```python
from build123d import *

# Parameters (mm, degrees)
SKETCH1_W            = 1180
SKETCH1_H            = 168
BASE_FLANGE1_DEPTH   = 12
EDGE_FLANGE1_START   = -590
EDGE_FLANGE1_DEPTH   = 1180
EDGE_FLANGE1_2_DEPTH = 1180


# Read off the part's stored shape, not the designer's step: Edge-Flange1
# Sheet-metal steps are written as plain solids
with BuildPart() as part:
    # Sketch1 → Base-Flange1 (new body)
    with BuildSketch(Plane(origin=(0, 0, 0), x_dir=(1, 0, 0), z_dir=(0, 1, 0))):
        Rectangle(SKETCH1_W, SKETCH1_H)
    extrude(amount=-BASE_FLANGE1_DEPTH)

    # Edge-Flange1 outline → Edge-Flange1 (cut)
    with BuildSketch(Plane.YZ.offset(EDGE_FLANGE1_START)):
        with BuildLine():
            Line((0, -84), (-8.382685902, -69.480762114))
            ThreePointArc((-8.382685902, -69.480762114), (-11.07999731, -62.968876332), (-12, -55.980762114))
            Line((-12, -55.980762114), (-12, -84))
            Line((-12, -84), (0, -84))
        make_face()
    extrude(amount=EDGE_FLANGE1_DEPTH, mode=Mode.SUBTRACT)

    # Edge-Flange1 2 outline → Edge-Flange1 2 (add)
    with BuildSketch(Plane.YZ.offset(EDGE_FLANGE1_START)):
        with BuildLine():
            Line((0, -55.980762114), (0, -84))
            Line((0, -84), (3, -89.196152423))
            Line((3, -89.196152423), (13.392304845, -83.196152423))
            Line((13.392304845, -83.196152423), (2.009618943, -63.480762114))
            ThreePointArc((2.009618943, -63.480762114), (0.511112606, -59.86304779), (0, -55.980762114))
        make_face()
    extrude(amount=EDGE_FLANGE1_2_DEPTH)


solid = part.part
```
Geometry check sheet. Reference: the model listing, model coordinates, mm. A direction names the side the tool comes from. Give positions to 0.01 mm unless a question says otherwise; leave off trailing zeros. Write each loop counter-clockwise with the first axis right and the second up, starting at its lowest first coordinate (ties: lowest second). Pieces come first, ordered by that corner, then holes.
1) Section check C-C, the plane y = 8.75. Record the boundary of the cut face in (x, z).
2) Access from +Z, -Z, +X, -X, +Y, -Y to the whole of each face (thin tool, end or side, straight path). Record for faces 1 (the flat face through (-8, 0, 13)), 2 (the flat face through (-8, -12, 13)).
3) Gauge pin test, flat ends, axial feed: pin 1 (5 mm diameter, centred on x = -184.5, y = 0.5, fed in from +Z); pin 2 (2 mm diameter, centred on x = -399, z = -34.5, fed in from +Y); pin 3 (3 mm diameter, centred on x = -280.5, y = 7.5, fed in from -Z). Record the tip position at first contact, or that the pin passes through.
4) Section check B-B, the plane z = 57. Record the boundary of the cut face in (x, y).
5) Material ranges on L1, parallel to Y at x = 530, z = 69; L2, parallel to Z at x = -482.5, y = 7; L3, parallel to Z at x = 65, y = 9.25, recorded low to high.
6) Section check A-A, the plane x = -275. Record the boundary of the cut face in (y, z), and give its area (3 significant figures).
Computed:
1. outline: (-590, -85.88) - (590, -85.88) - (590, -75.16) - (-590, -75.16) - close
2. face 1: +Z, +X, -X, +Y
2. face 2: +Z, -Z, +X, -X, -Y
3. pin 1: stops at z = 84
3. pin 2: stops at y = 0
3. pin 3: stops at z = -87.46
4. outline: (-590, -12) - (590, -12) - (590, 0) - (-590, 0) - close
5. L1: y = -12 to 0
5. L2: z = -86.89 to -72.12
5. L3: z = -85.59 to -76.02
6. outline: (-12, -55.98) arc R27 ccw to (-8.38, -69.48) - (3, -89.2) - (13.39, -83.2) - (2.01, -63.48) arc R15 cw to (0, -55.98) - (0, 84) - (-12, 84) - close
6. area: 2,080 mm2
